Check sheet for the modelled part. Datum: model origin and axes. Units: mm. Face numbers are marked on the shaded views. A direction names the side the tool comes from. Coordinates: 2 decimals unless noted, no trailing zeros. Loops run counter-clockwise (first coordinate to the right, second up) from the corner with the lowest first, then second, coordinate; pieces in that order, holes last. Notation, with made-up numbers: (-34, 85) - (5, 85) arc R9 cw to (5, 98) - close; hole circle Ø8 at (13, -14.75). An arc over 180 degrees is marked (long way). Use a Markdown table: item, result. Add a question column.
1) Go/stop test with flat-tipped pins: P1, Ø12, axis at x = 57, z = 12.5, coming from the +Y side; P2, Ø10.5, axis at x = 41.5, y = 53, coming from the +Z side; P3, Ø3, axis at x = 57.5, z = 16.5, coming from the -Y side; P4, Ø10, axis at x = 84.5, y = 29.5, coming from the +Z side. Record where each tip stops, or that it passes through.
2) Draft check along X on the marked faces 1, 2, 3 and 4. Enter one of: pulls with the +X half, pulls with the -X half, needs draft (parallel to the pull), parting line crosses it, or undercut.
3) Sectioned sample at A-A, the plane x = 50. State how many separate pieces and enclosed holes the cut face has, then the cut area to 3 significant figures.
4) Thickness scan on line 1 (Z direction, x = 30, y = 18); line 2 (Y direction, x = 50, z = 32.5); line 3 (Z direction, x = 39.5, y = 47.5). Record the ranges inside material, lowest first.
5) Sectioned sample at C-C, the plane z = 32. Enter the section's corners in (x, y).
6) Sectioned sample at D-D, the plane x = 24. Enter the section's corners in (y, z), then the cut area to 3 significant figures.
7) Tool access check on the marked faces 5, 6, 7, 8 and 9. Record the directions out of +Z, -Z, +X, -X, +Y, -Y that give a thin tool (end or side, any length) a straight path to the whole face; none if there is none.
8) Sectioned sample at B-B, the plane y = 37.5. Enter the section's corners in (x, z), then the cut area to 3 significant figures.
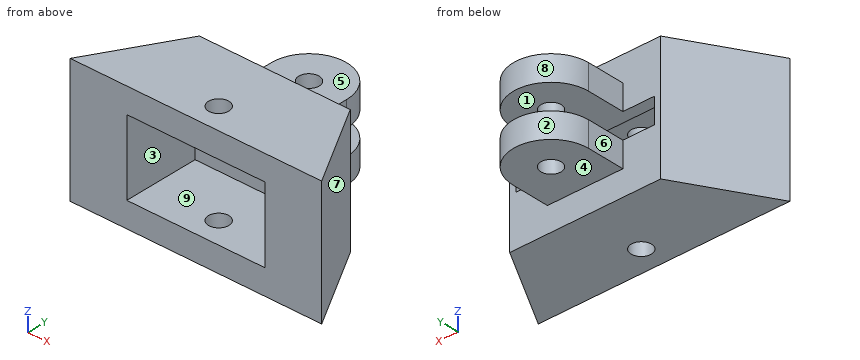
Autodesk Inventor part; units mm, degrees
ref_plane "YZ Plane" through (0, 0, 0) normal (1, 0, 0) x (0, 1, 0)
ref_plane "XZ Plane" through (0, 0, 0) normal (0, 1, 0) x (-1, 0, 0)
ref_plane "XY Plane" through (0, 0, 0) normal (0, 0, 1) x (1, 0, 0)
sketch "Sketch1" plane through (0, 0, 0) normal (0, 0, 1) x (1, 0, 0)
  line L0 (0, 0) -> (20, 34.641)
  line L1 (20, 34.641) -> (80, 34.641)
  line L2 (80, 34.641) -> (100, 0)
  line L3 (100, 0) -> (0, 0)
  dimension "d2" = 40
  dimension "d3" = 60
  dimension "d4" = 40
  dimension "d5" = 100
extrude "Extrusion1" add sketch "Sketch1" along normal blind 50
sketch "Sketch2" plane through (20, 34.641, 0) normal (0, 1, 0) x (1, 0, 0)
  line L0 (45, -10) -> (15, -10)
  line L1 (15, -10) -> (15, -40)
  line L2 (15, -40) -> (45, -40)
  line L3 (45, -40) -> (45, -10)
  line L4 (60, 0) -> (0, 0)
  line L5 (-20, 0) -> (-20, -50)
  line L6 (45, -20) -> (15, -20)
  line L7 (45, -30) -> (15, -30)
  point P0 (30, 0)
  point P1 (45, -25)
  point P2 (30, -40)
  dimension "d8" = 30
  dimension "d9" = 30
  dimension "d10" = 25
  dimension "d11" = 50
  dimension "d31" = 10
  dimension "d32" = 10
extrude "Extrusion2" add sketch "Sketch2" along normal blind 30 contours L3 L6 L1 L0 | L3 L2 L1 L7
sketch "Sketch3" plane through (0, 0, 0) normal (0, -1, 0) x (1, 0, 0)
  line L0 (22.5, 10) -> (77.5, 10)
  line L1 (77.5, 10) -> (77.5, 40)
  line L2 (77.5, 40) -> (22.5, 40)
  line L3 (22.5, 40) -> (22.5, 10)
  line L4 (0, 0) -> (0, 50)
  line L5 (0, 50) -> (100, 50)
  point P0 (50, 10)
  point P1 (22.5, 25)
  dimension "d14" = 55
  dimension "d15" = 30
  dimension "d16" = 50
  dimension "d17" = 25
extrude "Extrusion3" cut sketch "Sketch3" against normal blind 30
sketch "Sketch4" plane through (0, 0, 50) normal (0, 0, 1) x (1, 0, 0)
  circle A0 centre (50, 10) radius 4.05
  line L0 (0, 0) -> (100, 0)
  dimension "d20" = 8.1
  dimension "d21" = 10
  dimension "d22" = 50
extrude "Extrusion4" cut sketch "Sketch4" against normal up to surface (50 mm away)
sketch "Sketch5" plane through (35, 34.641, 40) normal (0, 0, 1) x (1, 0, 0)
  circle A0 centre (15, 15) radius 4.05
  line L0 (30, 0) -> (30, 30)
  line L1 (0, 30) -> (30, 30)
  line L2 (0, 0) -> (0, 30)
  arc A1 (30, 15) -> (0, 15) centre (15, 15) ccw
  line L3 (0, 15) -> (0, 30)
  line L4 (30, 30) -> (30, 15)
  line L5 (30, 30) -> (0, 30)
  point P0 (-35, -34.641)
  point P1 (15, 30)
  dimension "d25" = 8.1
  dimension "d26" = 15
  dimension "d27" = 15
  dimension "d28" = 15
extrude "Extrusion5" cut sketch "Sketch5" against normal up to surface (30 mm away)
sketch "Sketch6" plane through (0, 30, 0) normal (0, -1, 0) x (1, 0, 0)
  line L0 (77.5, 40) -> (77.5, 10)
  line L1 (22.5, 40) -> (77.5, 40)
  line L2 (22.5, 10) -> (22.5, 40)
  line L3 (77.5, 10) -> (22.5, 10)
  line L4 (77.5, 20) -> (22.5, 20)
  line L5 (22.5, 20) -> (22.5, 30)
  line L6 (22.5, 30) -> (77.5, 30)
  line L7 (77.5, 30) -> (77.5, 20)
  point P0 (0, 0)
  point P1 (22.5, 20)
  dimension "d33" = 10
  dimension "d34" = 10
extrude "Extrusion6" cut sketch "Sketch6" against normal up to surface (4.641 mm away) contours L0 L4 L2 L6
properties part number "center_wheel_well"
Solved:
| question | item | result |
|---|---|---|
| 1 | P1 | stops at y = 64.61 |
| 1 | P2 | stops at z = 40 |
| 1 | P3 | stops at y = 30 |
| 1 | P4 | stops at z = 50 |
| 2 | face 1 | undercut |
| 2 | face 2 | parting line crosses it |
| 2 | face 3 | undercut |
| 2 | face 4 | needs draft |
| 3 | separate pieces | 6 |
| 3 | enclosed holes | 0 |
| 3 | area | 1,060 mm2 |
| 4 | line 1 | z = 0 to 10, 40 to 50 |
| 4 | line 2 | y = 30 to 45.59, 53.69 to 64.64 |
| 4 | line 3 | z = 10 to 20, 30 to 40 |
| 5 | outline | (0, 0) - (22.5, 0) - (22.5, 30) - (77.5, 30) - (77.5, 0) - (100, 0) - (80, 34.64) - (65, 34.64) - (65, 49.64) arc R15 ccw to (35, 49.64) - (35, 34.64) - (20, 34.64) - close; hole circle Ø8.1 at (50, 49.64) |
| 6 | outline | (0, 0) - (34.64, 0) - (34.64, 20) - (30, 20) - (30, 10) - (0, 10) - close; (0, 40) - (30, 40) - (30, 30) - (34.64, 30) - (34.64, 50) - (0, 50) - close |
| 6 | area | 786 mm2 |
| 7 | face 5 | +Z, +X, -X, +Y |
| 7 | face 6 | +Z, -Z, -X, +Y |
| 7 | face 7 | +Z, -Z, +X, +Y |
| 7 | face 8 | +Z, -Z, +Y |
| 7 | face 9 | -Y |
| 8 | outline | (35, 10) - (65, 10) - (65, 20) - (35, 20) - close; (35, 30) - (65, 30) - (65, 40) - (35, 40) - close |
| 8 | area | 600 mm2 |
